The model under review builds one solid part; all positions refer to its coordinate system, in mm. Face numbers are marked on the shaded views. Give positions to 0.01 mm unless a question says otherwise; leave off trailing zeros. Loops run counter-clockwise (first coordinate to the right, second up) from the corner with the lowest first, then second, coordinate; pieces in that order, holes last. Notation, with made-up numbers: M 35.25,29.5 L 56.25,29.5 A28 cw 56.25,48.5 Z; hole C 82.25,31.25 d8. An arc over 180 degrees is marked long. Return JSON: item names as keys, results as strings.
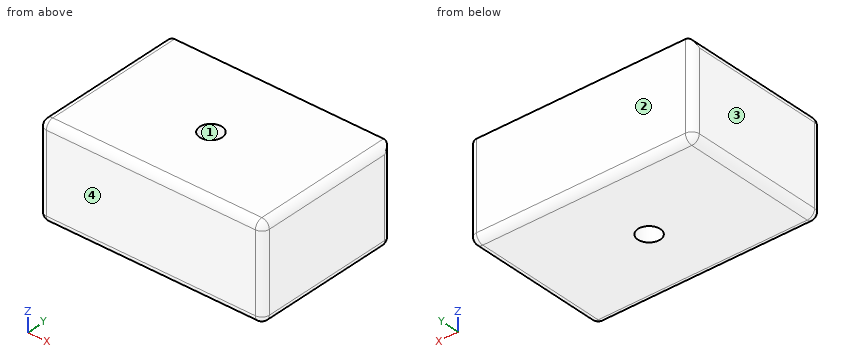
```python
from build123d import *

# Parameters (mm, degrees)
F0_W         = 300
F0_H         = 200
F0_R         = 15
F1_DEPTH     = 25
F2_DEPTH     = 100
F3_R         = 10
F6_T1_DEPTH  = 105
F6_T3_DEPTH  = 180
F6_T5_DEPTH  = 130
F6_T7_DEPTH  = 280
F6_T9_DEPTH  = 140
F6_T11_DEPTH = 215
F6_S15_W     = 10.2
F6_S15_H     = 10.2
F6_T16_DEPTH = 10.2
F6_S21_W     = 10.2
F6_S21_H     = 10.2
F6_T22_DEPTH = 10.2
F6_S27_W     = 10.2
F6_S27_H     = 10.2
F6_T28_DEPTH = 10.2
F6_S33_W     = 10.2
F6_S33_H     = 10.2
F6_T34_DEPTH = 10.2
F6_S39_W     = 10.2
F6_S39_H     = 10.2
F6_T40_DEPTH = 10.2
F6_T44_ANGLE = 90


# Not quite as in the source:
# - a fillet or chamfer that OpenCascade refuses, or shapes differently, is made with other operations: its cross-section is extruded or revolved along the edge and cut away or added
# - a feature of the source that left no trace in its solid (it failed there, or was rolled back) is left out


with BuildPart() as f1:
    # F0 (on Top) → F1 (new body)
    with BuildSketch(Plane.XY):
        with Locations((-0.7391218096, 3.9163683355)):
            Rectangle(F0_W, F0_H)
        with Locations((-1.9179330509, -1.0798395535)):
            Circle(F0_R, mode=Mode.SUBTRACT)
    extrude(amount=F1_DEPTH)

    # F0 (on Top) → F2 (join)
    with BuildSketch(Plane.XY):
        with Locations((-0.7391218096, 3.9163683355)):
            Rectangle(F0_W, F0_H)
        with Locations((-1.9179330509, -1.0798395535)):
            Circle(F0_R, mode=Mode.SUBTRACT)
    extrude(amount=-F2_DEPTH)

    # F3
    f3_edges = [f1.edges().sort_by_distance(p)[0] for p in [
        (-150.739122, 3.916368, 25),
    ]]
    fillet(f3_edges, radius=F3_R)

    # F6: fillet of radius 10 on 11 edges, made by hand

    # F6_s2 → F6_t1 (cut)
    with BuildSketch(Plane.XY.offset(-90)):
        with BuildLine():
            ThreePointArc((-150.7391218096, -86.0836316645), (-147.8101896215, -93.1546994763), (-140.7391218096, -96.0836316645))
            Line((-140.7391218096, -96.0836316645), (-150.7391218096, -96.0836316645))
            Line((-150.7391218096, -96.0836316645), (-150.7391218096, -86.0836316645))
        make_face()
        with BuildLine():
            ThreePointArc((139.2608781904, -96.0836316645), (146.3319460023, -93.1546994763), (149.2608781904, -86.0836316645))
            Line((149.2608781904, -86.0836316645), (149.2608781904, -96.0836316645))
            Line((149.2608781904, -96.0836316645), (139.2608781904, -96.0836316645))
        make_face()
    extrude(amount=F6_T1_DEPTH, mode=Mode.SUBTRACT)

    # F6_s4 → F6_t3 (cut)
    with BuildSketch(Plane.XZ.offset(-93.9163683355)):
        with BuildLine():
            ThreePointArc((-150.7391218096, -90), (-147.8101896215, -97.0710678119), (-140.7391218096, -100))
            Line((-140.7391218096, -100), (-150.7391218096, -100))
            Line((-150.7391218096, -100), (-150.7391218096, -90))
        make_face()
        with BuildLine():
            ThreePointArc((139.2608781904, -100), (146.3319460023, -97.0710678119), (149.2608781904, -90))
            Line((149.2608781904, -90), (149.2608781904, -100))
            Line((149.2608781904, -100), (139.2608781904, -100))
        make_face()
    extrude(amount=F6_T3_DEPTH, mode=Mode.SUBTRACT)

    # F6_s6 → F6_t5 (cut)
    with BuildSketch(Plane.XY.offset(-90)):
        with BuildLine():
            ThreePointArc((-150.7391218096, 93.9163683355), (-147.8101896215, 100.9874361474), (-140.7391218096, 103.9163683355))
            Line((-140.7391218096, 103.9163683355), (-150.7391218096, 103.9163683355))
            Line((-150.7391218096, 103.9163683355), (-150.7391218096, 93.9163683355))
        make_face()
    extrude(amount=F6_T5_DEPTH, mode=Mode.SUBTRACT)

    # F6_s8 → F6_t7 (cut)
    with BuildSketch(Plane.YZ.offset(-140.7391218096)):
        with BuildLine():
            ThreePointArc((-96.0836316645, -90), (-93.1546994763, -97.0710678119), (-86.0836316645, -100))
            Line((-86.0836316645, -100), (-96.0836316645, -100))
            Line((-96.0836316645, -100), (-96.0836316645, -90))
        make_face()
        with BuildLine():
            ThreePointArc((-96.0836316645, 15), (-93.1546994763, 22.0710678119), (-86.0836316645, 25))
            Line((-86.0836316645, 25), (-96.0836316645, 25))
            Line((-96.0836316645, 25), (-96.0836316645, 15))
        make_face()
        with BuildLine():
            ThreePointArc((93.9163683355, -100), (100.9874361474, -97.0710678119), (103.9163683355, -90))
            Line((103.9163683355, -90), (103.9163683355, -100))
            Line((103.9163683355, -100), (93.9163683355, -100))
        make_face()
    extrude(amount=F6_T7_DEPTH, mode=Mode.SUBTRACT)

    # F6_s10 → F6_t9 (cut)
    with BuildSketch(Plane.XY.offset(-90)):
        with BuildLine():
            ThreePointArc((139.2608781904, 103.9163683355), (146.3319460023, 100.9874361474), (149.2608781904, 93.9163683355))
            Line((149.2608781904, 93.9163683355), (149.2608781904, 103.9163683355))
            Line((149.2608781904, 103.9163683355), (139.2608781904, 103.9163683355))
        make_face()
    extrude(amount=F6_T9_DEPTH, mode=Mode.SUBTRACT)

    # F6_s12 → F6_t11 (cut)
    with BuildSketch(Plane.XZ.offset(-128.9163683355)):
        with BuildLine():
            ThreePointArc((139.2608781904, 25), (146.3319460023, 22.0710678119), (149.2608781904, 15))
            Line((149.2608781904, 15), (149.2608781904, 25))
            Line((149.2608781904, 25), (139.2608781904, 25))
        make_face()
    extrude(amount=F6_T11_DEPTH, mode=Mode.SUBTRACT)


with BuildPart() as f6_tool14:
    # F6_s15 → F6_t16 (new body)
    with BuildSketch(Plane.YZ.offset(-140.7391218096)):
        with Locations((-91.1836316645, -95.1)):
            Rectangle(F6_S15_W, F6_S15_H)
    extrude(amount=-F6_T16_DEPTH)

    # F6_s17 → F6_t18 (revolve, cut)
    with BuildSketch(Plane(origin=(-140.7391218096, -86.0836316645, -90), x_dir=(0, 0.7071067812, 0.7071067812), z_dir=(0, -0.7071067812, 0.7071067812))):
        with BuildLine():
            ThreePointArc((0, -10), (10, 0), (0, 10))
            Line((0, 10), (0, -10))
        make_face()
    revolve(axis=Axis((-140.7391218096, -86.0836316645, -90), (-1, 0, 0)), mode=Mode.SUBTRACT)


with BuildPart() as f1_1:
    add(f1.part)

    # F6_t13: cut F6_tool14
    add(f6_tool14.part, mode=Mode.SUBTRACT)


with BuildPart() as f6_tool20:
    # F6_s21 → F6_t22 (new body)
    with BuildSketch(Plane.YZ.offset(-140.7391218096)):
        with Locations((99.0163683355, -95.1)):
            Rectangle(F6_S21_W, F6_S21_H)
    extrude(amount=-F6_T22_DEPTH)

    # F6_s23 → F6_t24 (revolve, cut)
    with BuildSketch(Plane(origin=(-140.7391218096, 93.9163683355, -90), x_dir=(0, -0.7071067812, 0.7071067812), z_dir=(0, -0.7071067812, -0.7071067812))):
        with BuildLine():
            ThreePointArc((0, -10), (10, 0), (0, 10))
            Line((0, 10), (0, -10))
        make_face()
    revolve(axis=Axis((-140.7391218096, 93.9163683355, -90), (-1, 0, 0)), mode=Mode.SUBTRACT)


with BuildPart() as f1_2:
    add(f1_1.part)

    # F6_t19: cut F6_tool20
    add(f6_tool20.part, mode=Mode.SUBTRACT)


with BuildPart() as f6_tool26:
    # F6_s27 → F6_t28 (new body)
    with BuildSketch(Plane.XZ.offset(86.0836316645)):
        with Locations((144.3608781904, -95.1)):
            Rectangle(F6_S27_W, F6_S27_H)
    extrude(amount=F6_T28_DEPTH)

    # F6_s29 → F6_t30 (revolve, cut)
    with BuildSketch(Plane(origin=(139.2608781904, -86.0836316645, -90), x_dir=(-0.7071067812, 0, 0.7071067812), z_dir=(0.7071067812, 0, 0.7071067812))):
        with BuildLine():
            ThreePointArc((0, -10), (10, 0), (0, 10))
            Line((0, 10), (0, -10))
        make_face()
    revolve(axis=Axis((139.2608781904, -86.0836316645, -90), (0, -1, 0)), mode=Mode.SUBTRACT)


with BuildPart() as f1_3:
    add(f1_2.part)

    # F6_t25: cut F6_tool26
    add(f6_tool26.part, mode=Mode.SUBTRACT)


with BuildPart() as f6_tool32:
    # F6_s33 → F6_t34 (new body)
    with BuildSketch(Plane.XZ.offset(86.0836316645)):
        with Locations((144.3608781904, 20.1)):
            Rectangle(F6_S33_W, F6_S33_H)
    extrude(amount=F6_T34_DEPTH)

    # F6_s35 → F6_t36 (revolve, cut)
    with BuildSketch(Plane(origin=(139.2608781904, -86.0836316645, 15), x_dir=(-0.7071067812, 0, -0.7071067812), z_dir=(-0.7071067812, 0, 0.7071067812))):
        with BuildLine():
            ThreePointArc((0, -10), (10, 0), (0, 10))
            Line((0, 10), (0, -10))
        make_face()
    revolve(axis=Axis((139.2608781904, -86.0836316645, 15), (0, -1, 0)), mode=Mode.SUBTRACT)


with BuildPart() as f1_4:
    add(f1_3.part)

    # F6_t31: cut F6_tool32
    add(f6_tool32.part, mode=Mode.SUBTRACT)


with BuildPart() as f6_tool38:
    # F6_s39 → F6_t40 (new body)
    with BuildSketch(Plane.XY.offset(-90)):
        with Locations((144.3608781904, 99.0163683355)):
            Rectangle(F6_S39_W, F6_S39_H)
    extrude(amount=-F6_T40_DEPTH)

    # F6_s41 → F6_t42 (revolve, cut)
    with BuildSketch(Plane(origin=(139.2608781904, 93.9163683355, -90), x_dir=(-0.7071067812, -0.7071067812, 0), z_dir=(0.7071067812, -0.7071067812, 0))):
        with BuildLine():
            ThreePointArc((0, -10), (10, 0), (0, 10))
            Line((0, 10), (0, -10))
        make_face()
    revolve(axis=Axis((139.2608781904, 93.9163683355, -90), (0, 0, -1)), mode=Mode.SUBTRACT)


with BuildPart() as f1_5:
    add(f1_4.part)

    # F6_t37: cut F6_tool38
    add(f6_tool38.part, mode=Mode.SUBTRACT)

    # F6_s43 → F6_t44 (revolve, cut)
    with BuildSketch(Plane.XY.offset(15)):
        with BuildLine():
            ThreePointArc((-140.7391218096, -96.0836316645), (-147.8101896215, -93.1546994763), (-150.7391218096, -86.0836316645))
            Line((-150.7391218096, -86.0836316645), (-150.7391218096, -96.0836316645))
            Line((-150.7391218096, -96.0836316645), (-140.7391218096, -96.0836316645))
        make_face()
    revolve(axis=Axis((-140.7391218096, -96.0836316645, 15), (0, 1, 0)), revolution_arc=F6_T44_ANGLE, mode=Mode.SUBTRACT)


solid = f1_5.part
```
1) The part is to be moulded in two halves that separate along Y. For the marked faces 1, 2, 3 and 4, say which applies: released by +Y, released by -Y, zero draft, split by the parting line, or undercut.
From the geometry:
{"face 1": "undercut", "face 2": "released by +Y", "face 3": "zero draft", "face 4": "released by -Y"}
2) Wall thickness on L1, parallel to X at y = 3.5, z = 16.5; L2, parallel to X at y = 94.5, z = -15.5; L3, parallel to X at y = 20, z = -92: over which ranges is each line inside the solid? List them lowest first. Write a range as from..to.
From the geometry:
{"L1": "-150.63..-16.2, 12.37..149.15", "L2": "-150.72..149.24", "L3": "-150.54..149.06"}
3) Consider section A-A on y = -10. Write out the cut boundary in (x, z).
From the geometry:
{"outline": "M -150.74,-90 A10 ccw -140.74,-100 L -13.98,-100 L -13.98,25 L -140.74,25 A10 ccw -150.74,15 Z; M 10.14,-100 L 139.26,-100 A10 ccw 149.26,-90 L 149.26,15 A10 ccw 139.26,25 L 10.14,25 Z"}
4) Consider section B-B on x = -12. Write out the cut boundary in (y, z), then the cut area to 3 significant figures.
From the geometry:
{"outline": "M -96.08,-90 A10 ccw -86.08,-100 L -12.19,-100 L -12.19,25 L -86.08,25 A10 ccw -96.08,15 Z; M 10.03,-100 L 93.92,-100 A10 ccw 103.92,-90 L 103.92,25 L 10.03,25 Z", "area": "22,200 mm²"}
